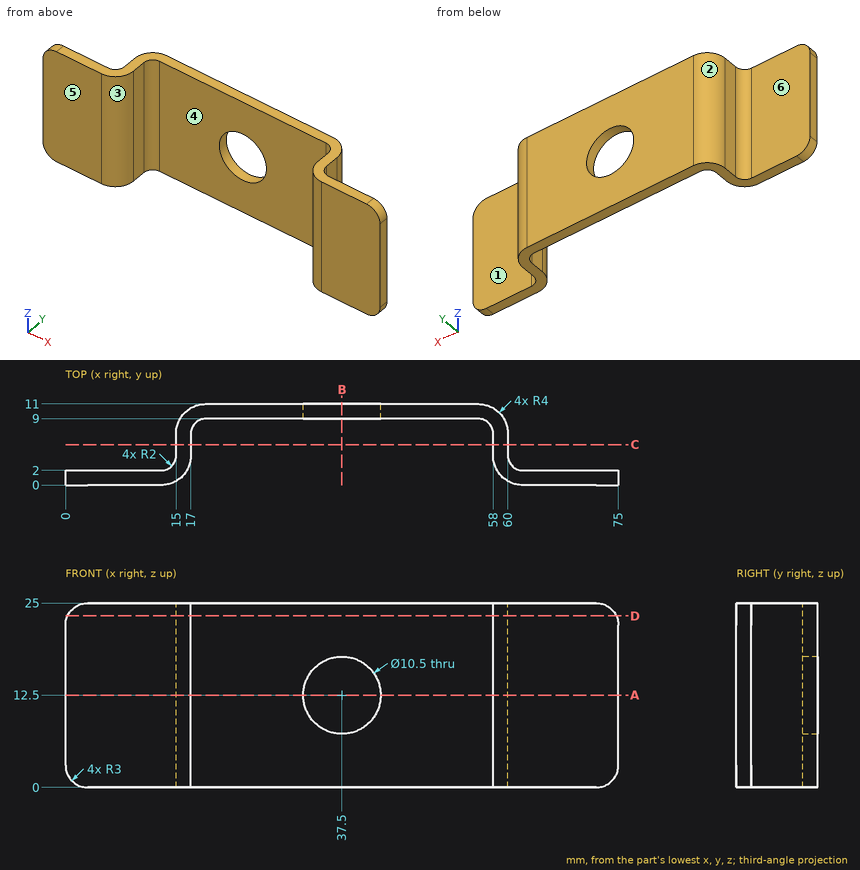
Geometry check sheet. Reference: drawing and pictorial views, mm from the part's lowest x, y, z. A direction names the side the tool comes from. Give positions to 0.01 mm unless a question says otherwise; leave off trailing zeros. Order: outer loops, then holes, each group sorted by start corner. A loop starts at its lowest first (then second) coordinate and runs counter-clockwise, first axis right, second up. Notation, with made-up numbers: (-3.5, 39.25) -> (38.5, 39.25) arc R26 cw to (38.5, 54.25) -> close; hole circle Ø9 at (64.25, 29.5). An arc over 180 degrees is marked (long way). Use CSV: the item, a comma, the result in double quotes. Start each with the question number.
1) Material ranges on line 1 (X direction, y = 7.25, z = 19); line 2 (Y direction, x = 23.5, z = 3); line 3 (X direction, y = 10.4, z = 12.5), recorded low to high. Write a range as from..to.
2) Go/stop test with flat-tipped pins: P1, Ø1.5, axis at y = 5, z = 6.5, coming from the +X side; P2, Ø1, axis at x = 15.5, z = 15, coming from the -Y side; P3, Ø0.9, axis at y = 5, z = 7, coming from the -X side. Record where each tip stops, or that it passes through.
3) Sectioned sample at D-D, the plane z = 23.25. Record the boundary of the cut face in (x, y).
4) Sectioned sample at A-A, the plane z = 12.5. Record the boundary of the cut face in (x, y), plus the area to 3 significant figures.
5) Mould release check, pull along X, two halves, no side actions. Record for the marked faces 1, 2, 3 and 4: released by +X, released by -X, zero draft, split by the parting line, or undercut.
6) Sectioned sample at C-C, the plane y = 5.5. Record the boundary of the cut face in (x, z).
7) Sectioned sample at B-B, the plane x = 37.5. Record the boundary of the cut face in (y, z).
8) Set-up check for the marked faces 5 and 6: record each of +Z, -Z, +X, -X, +Y, -Y from which the full face is reachable in a straight line by a thin tool's end or side.
Recorded:
1,line 1,"15.01..17.02, 57.98..59.99"
1,line 2,"9..11"
1,line 3,"16.89..32.25, 42.75..58.11"
2,P1,"x = 60"
2,P2,"y = 0.54"
2,P3,"x = 15"
3,outline,"(0.27, 0) -> (13, 0) arc R4 ccw to (17, 4) -> (17, 7) arc R2 cw to (19, 9) -> (56, 9) arc R2 cw to (58, 7) -> (58, 4) arc R4 ccw to (62, 0) -> (74.73, 0) -> (74.73, 2) -> (62, 2) arc R2 cw to (60, 4) -> (60, 7) arc R4 ccw to (56, 11) -> (19, 11) arc R4 ccw to (15, 7) -> (15, 4) arc R2 cw to (13, 2) -> (0.27, 2) -> close"
4,outline,"(0, 0) -> (13, 0) arc R4 ccw to (17, 4) -> (17, 7) arc R2 cw to (19, 9) -> (32.25, 9) -> (32.25, 11) -> (19, 11) arc R4 ccw to (15, 7) -> (15, 4) arc R2 cw to (13, 2) -> (0, 2) -> close; (42.75, 9) -> (56, 9) arc R2 cw to (58, 7) -> (58, 4) arc R4 ccw to (62, 0) -> (75, 0) -> (75, 2) -> (62, 2) arc R2 cw to (60, 4) -> (60, 7) arc R4 ccw to (56, 11) -> (42.75, 11) -> close"
4,area,"155 mm2"
5,face 1,"zero draft"
5,face 2,"released by -X"
5,face 3,"undercut"
5,face 4,"undercut"
6,outline,"(15, 0) -> (17, 0) -> (17, 25) -> (15, 25) -> close; (58, 0) -> (60, 0) -> (60, 25) -> (58, 25) -> close"
7,outline,"(9, 0) -> (11, 0) -> (11, 7.25) -> (9, 7.25) -> close; (9, 17.75) -> (11, 17.75) -> (11, 25) -> (9, 25) -> close"
8,face 5,"+Z, -Z, +X, -X, -Y"
8,face 6,"+Z, -Z, -X, +Y"
